Can you work these out from the model? Positions are in its coordinate system, mm. A direction names the side the tool comes from. Round coordinates to 2 decimals unless told otherwise and drop trailing zeros. Loops run counter-clockwise (first coordinate to the right, second up) from the corner with the lowest first, then second, coordinate; pieces in that order, holes last. Notation, with made-up numbers: M 60,-9.5 L 99,-9.5 A16 ccw 99,5.5 Z; hole C 73.25,78.25 d1. An arc over 180 degrees is marked long. Return JSON: item names as keys, results as strings.
Autodesk Inventor part; units mm, degrees
ref_plane "YZ Plane" through (0, 0, 0) normal (1, 0, 0) x (0, 1, 0)
ref_plane "XZ Plane" through (0, 0, 0) normal (0, 1, 0) x (-1, 0, 0)
ref_plane "XY Plane" through (0, 0, 0) normal (0, 0, 1) x (1, 0, 0)
sketch "Sketch1" plane through (0, 0, 0) normal (0, 0, 1) x (1, 0, 0)
  line L0 (-10, -15) -> (10, -15)
  line L1 (10, -15) -> (10, 15)
  line L2 (10, 15) -> (-10, 15) construction
  line L3 (-10, 19.4339) -> (-10, -15)
  line L4 (-10, -15) -> (10, 15) construction
  line L5 (10, -15) -> (-10, 15) construction
  line L6 (10, 15) -> (22.6785, 42.1892)
  line L7 (22.6785, 42.1892) -> (4.5524, 50.6416) construction
  line L8 (6.4262, 54.6601) -> (-10, 19.4339)
  line L9 (9.8228, 57.5101) -> (22.6785, 42.1892) construction
  line L10 (22.6785, 42.1892) -> (45.6599, 61.4729)
  line L11 (45.6599, 61.4729) -> (32.8041, 76.7938)
  line L12 (32.8041, 76.7938) -> (6.4262, 54.6601)
  line L13 (12.6785, 27.1892) -> (32.6785, 57.1892) construction
  line L14 (32.6785, 27.1892) -> (12.6785, 57.1892) construction
  point P0 (0, 0)
  dimension "d3" = 30
  dimension "d4" = 20
  dimension "d5" = 30
  dimension "d6" = 34.4339
  dimension "d9" = 90
  dimension "d10" = 20
  dimension "d12" = 155
  dimension "d13" = 35.2262
  dimension "d14" = 22.1337
  dimension "d15" = 26.3779
  dimension "d16" = 20
extrude "Extrusion1" add sketch "Sketch1" along normal blind 20
shell "Shell1" thickness 2 removed faces 2 at (-3.3333, -15, 6.6667) at (41.3746, 66.5798, 6.6667)
properties part number "bent_finger_model"
Q1. If I drill on line 1 along X through (y, z) = (3.5, 5.5); line 2 along Z through (x, y) = (16.5, 59); line 3 along X through (y, z) = (18, 10.5), over which ranges is the centre line in solid material (lowest first)?
Results:
{"line 1": "x = -10 to -8, 8 to 10", "line 2": "z = 0 to 2, 18 to 20", "line 3": "x = -10 to -8, 9.19 to 11.4"}
Q2. Suppose I cut it at B-B, the plane z = 12. Please give me the cut outline in (x, y), plus the area to 3 significant figures.
Results:
{"outline": "M -10,-15 L -8,-15 L -8,18.99 L 8.05,53.41 L 34.09,75.26 L 32.8,76.79 L 6.43,54.66 L -10,19.43 Z; M 8,-15 L 10,-15 L 10,15 L 22.68,42.19 L 45.66,61.47 L 44.37,63 L 21.05,43.44 L 8,15.44 Z", "area": "395 mm2"}
Q3. Thinking about a two-plate mould opening in X: for faces 1 (the flat face through (12, 30, 18)), 2 (the flat face through (11, 32, 20)), 3 (the flat face through (-1.672, 37.294, 9.86)), which applies, pulls with the +X half, pulls with the -X half, needs draft (parallel to the pull), parting line crosses it, or undercut?
Results:
{"face 1": "undercut", "face 2": "needs draft", "face 3": "pulls with the -X half"}
Q4. Suppose I cut it at D-D, the plane y = 57.5. Please give me the cut outline in (x, z).
Results:
{"outline": "M 9.81,0 L 40.93,0 L 40.93,20 L 9.81,20 Z; hole M 12.92,2 L 37.81,2 L 37.81,18 L 12.92,18 Z"}
Q5. On a 3-axis mill with a long thin cutter (end or side, diameter ignored), from which of +Z, -Z, +X, -X, +Y, -Y can I reach the whole of each face in a straight line? I mean faces 4 (the flat face through (10, 0, 10)), 5 (the flat face through (21.25, 64.49, 9.89)), 6 (the flat face through (8, 0, 10)). Say none if no direction works.
Results:
{"face 4": "+Z, -Z, +X, -Y", "face 5": "none", "face 6": "-Y"}
Q6. Suppose I cut it at C-C, the plane x = 35. Please give me the cut outline in (y, z), plus the area to 3 significant figures.
Results:
{"outline": "M 52.53,0 L 74.18,0 L 74.18,2 L 55.14,2 L 55.14,18 L 74.18,18 L 74.18,20 L 52.53,20 Z", "area": "128 mm2"}
Q7. I'm going to push flat-ended pins straight in: pin 1 Ø10 at (y, z) = (28.5, 4.5) entering from +X; pin 2 Ø1.5 at (y, z) = (13.5, 16.5) entering from +X; pin 3 Ø1 at (x, z) = (20, 9) entering from -Y. Where does each tip first touch, or does it pass through?
Results:
{"pin 1": "stops at x = 18.63", "pin 2": "stops at x = 10", "pin 3": "stops at y = 35.37"}
Q8. Suppose I cut it at A-A, the plane y = -3. Please give me the cut outline in (x, z).
Results:
{"outline": "M -10,0 L 10,0 L 10,20 L -10,20 Z; hole M -8,2 L 8,2 L 8,18 L -8,18 Z"}
